from build123d import *

# Parameters (mm, degrees)
BOSS_EXTRUDE1_DEPTH = 9
BOSS_EXTRUDE4_DEPTH = 1
SKETCH2_R           = 2.5
BOSS_EXTRUDE2_DEPTH = 5
CHAMFER2_SIZE       = 0.5


with BuildPart() as part:
    # Sketch1 → Boss-Extrude1 (new body)
    with BuildSketch(Plane(origin=(0, 0, 0), x_dir=(1, 0, 0), z_dir=(0, 1, 0))):
        with BuildLine():
            Line((0, 20.4), (0, 0))
            Line((0, 0), (30.8, 0))
            Line((30.8, 0), (30.8, 20.4))
            ThreePointArc((30.8, 20.4), (15.4, 31.319313711), (0, 20.4))
        make_face()
        with BuildLine():
            ThreePointArc((10.8, 15.3), (9.3, 20.4), (10.8, 25.5))
            Line((10.8, 25.5), (20, 25.5))
            ThreePointArc((20, 25.5), (21.5, 20.4), (20, 15.3))
            Line((20, 15.3), (10.8, 15.3))
        make_face(mode=Mode.SUBTRACT)
    extrude(amount=BOSS_EXTRUDE1_DEPTH)

    # Sketch6 → Boss-Extrude4 (add, symmetric)
    with BuildSketch(Plane(origin=(15.4, 0, 0), x_dir=(0, 0, -1), z_dir=(1, 0, 0))):
        Polygon((15.3, 9), (15.3, 12), (17.3, 12), (13.8, 14.020725942), (13.8, 9), align=None)
        Polygon((25.5, 9), (25.5, 12), (23.5, 12), (27, 14.020725942), (27, 9), align=None)
    extrude(amount=BOSS_EXTRUDE4_DEPTH, both=True)

    # Sketch2 → Boss-Extrude2 (add)
    with BuildSketch(Plane.XY):
        with Locations(Location((10.4, 4.5, 0), (0, 0, 180))):
            Circle(SKETCH2_R)
        with Locations(Location((20.4, 4.5, 0), (0, 0, 180))):
            Circle(SKETCH2_R)
    extrude(amount=BOSS_EXTRUDE2_DEPTH)

    # Chamfer2
    chamfer2_edges = [part.edges().sort_by_distance(p)[0] for p in [
        (14.4, 9, -14.55),
        (15.4, 9, -13.8),
        (16.4, 9, -14.55),
        (14.4, 9, -26.25),
        (15.4, 9, -27),
        (16.4, 9, -26.25),
    ]]
    chamfer(chamfer2_edges, length=CHAMFER2_SIZE)


solid = part.part
Geometry check sheet. Reference: the model listing, model coordinates, mm. A direction names the side the tool comes from. Round coordinates to 2 decimals unless told otherwise and drop trailing zeros. Order: outer loops, then holes, each group sorted by start corner. A loop starts at its lowest first (then second) coordinate and runs counter-clockwise, first axis right, second up. Notation, with made-up numbers: M -8.5,10.5 L -4.5,10.5 A14 cw -4.5,28.5 Z; hole C -2.75,44.5 d8. An arc over 180 degrees is marked long. Write each question's results on one line, items separated by ' | '. Start each with the question number.
1. Cross-section at A-A on y = 1. Record the boundary of the cut face in (x, z), plus the area to 3 significant figures.
2. Cross-section at C-C on y = 5.5. Record the boundary of the cut face in (x, z).
3. Cross-section at B-B on x = 16. Record the boundary of the cut face in (y, z).
4. Draft check along X on faces 4 (the face through (15.41, 13, -25.23)), 5 (the face through (14.4, 12, -15)), 6 (the face through (16.4, 12, -26)), 7 (the face through (22.24, 2.81, 2.46)). Enter one of: pulls with the +X half, pulls with the -X half, needs draft (parallel to the pull), parting line crosses it, or undercut.
5. Go/stop test with flat-tipped pins: P1, Ø2, axis at x = 15.5, y = 12.5, coming from the +Z side; P2, Ø4.5, axis at x = 14.5, y = 7, coming from the +Z side; P3, Ø2, axis at x = 15.5, y = 12, coming from the -Z side; P4, Ø4, axis at y = 12, z = -11.5, coming from the -X side. Record where each tip stops, or that it passes through.
6. Set-up check for faces 1 (the face through (9.3, 4.4, -20.3)), 2 (the face through (15, 5, -15.3)), 3 (the face through (12.24, 2.81, 2.46)): record each of +Z, -Z, +X, -X, +Y, -Y from which the full face is reachable in a straight line by a thin tool's end or side.
7. Cross-section at D-D on z = -7. Record the boundary of the cut face in (x, y), plus the area to 3 significant figures.
8. Material ranges on L1, parallel to X at y = 4.5, z = 1; L2, parallel to Y at x = 17, z = -1; L3, parallel to X at y = 1.25, z = -23, recorded low to high. Write a range as from..to.
Resolved:
1) outline: M 0,-20.4 A16.32 ccw 30.8,-20.4 L 30.8,0 L 0,0 Z; hole M 10.8,-25.5 L 20,-25.5 A9.42 ccw 20,-15.3 L 10.8,-15.3 A9.42 ccw Z | area: 759 mm2
2) outline: M 0,-20.4 A16.32 ccw 30.8,-20.4 L 30.8,0 L 22.69,0 L 22.69,5 L 18.11,5 L 18.11,0 L 12.69,0 L 12.69,5 L 8.11,5 L 8.11,0 L 0,0 Z; hole M 10.8,-25.5 L 20,-25.5 A9.42 ccw 20,-15.3 L 10.8,-15.3 A9.42 ccw Z
3) outline: M 0,-31.31 L 9,-31.31 L 9,-27.5 L 9.5,-27 L 14.02,-27 L 12,-23.5 L 12,-25.5 L 0,-25.5 Z; M 0,-15.3 L 12,-15.3 L 12,-17.3 L 14.02,-13.8 L 9.5,-13.8 L 9,-13.3 L 9,0 L 0,0 Z
4) face 4: needs draft | face 5: pulls with the -X half | face 6: pulls with the +X half | face 7: undercut
5) P1: z = -13.8 | P2: z = 0 | P3: z = -27 | P4: through
6) face 1: +Y, -Y | face 2: -Y | face 3: +Z
7) outline: M 0,0 L 30.8,0 L 30.8,9 L 0,9 Z | area: 277 mm2
8) L1: 7.9..12.9, 17.9..22.9 | L2: 0..9 | L3: 1.18..9.67, 21.13..29.62
